Could you check a few things on this drawing? It's one solid part, dimensions in mm from its lowest x, y, z. A direction names the side the tool comes from. Coordinates: 2 decimals unless noted, no trailing zeros. Write each loop counter-clockwise with the first axis right and the second up, starting at its lowest first coordinate (ties: lowest second). Pieces come first, ordered by that corner, then holes.
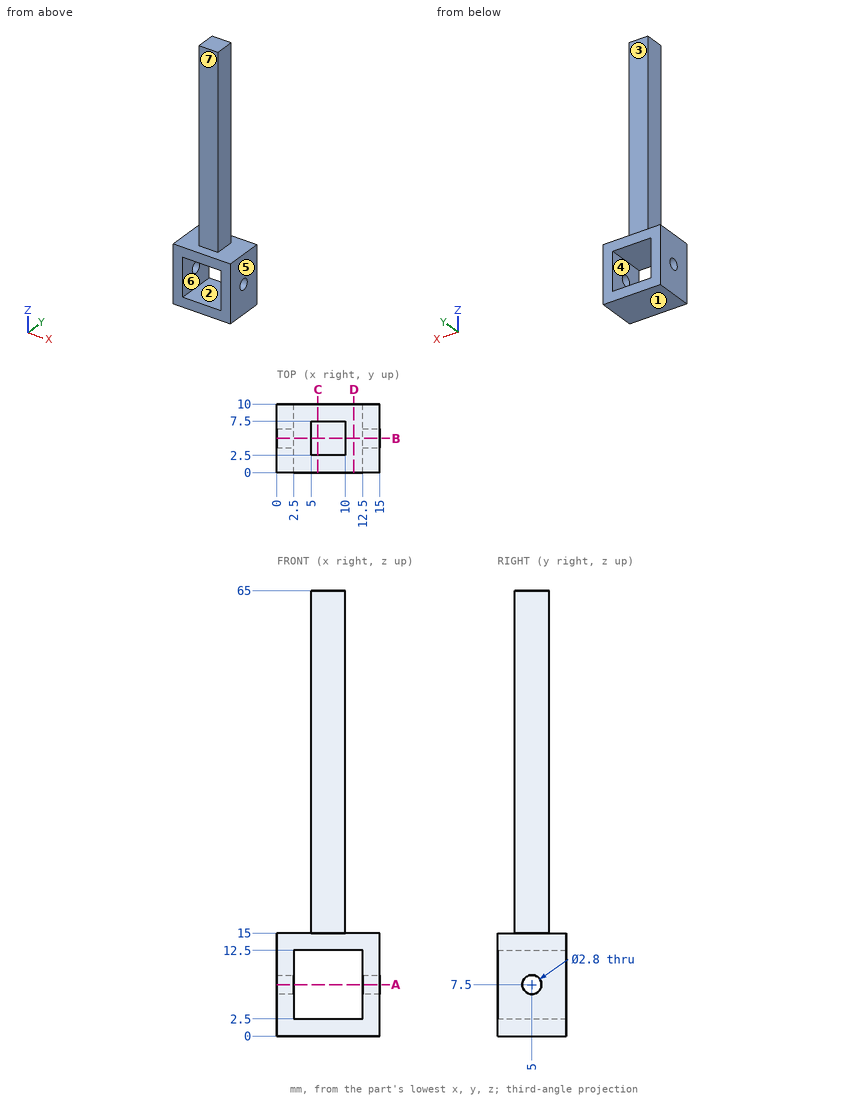
1) Imagine slicing it at A-A on z = 7.5. Please give me the cut outline in (x, y), then the cut area to 3 significant figures.
Values follow:
outline: (0, 0) - (2.5, 0) - (2.5, 3.6) - (0, 3.6) - close; (0, 6.4) - (2.5, 6.4) - (2.5, 10) - (0, 10) - close; (12.5, 0) - (15, 0) - (15, 3.6) - (12.5, 3.6) - close; (12.5, 6.4) - (15, 6.4) - (15, 10) - (12.5, 10) - close
area: 36.0 mm2
2) We'd pull the mould along Z, two halves only. Please class the marked faces 1, 2, 3 and 4: pulls with the +Z half, pulls with the -Z half, needs draft (parallel to the pull), parting line crosses it, or undercut.
Values follow:
face 1: pulls with the -Z half
face 2: undercut
face 3: needs draft
face 4: undercut
3) Imagine slicing it at B-B on y = 5. Please give me the cut outline in (x, z).
Values follow:
outline: (0, 0) - (15, 0) - (15, 6.1) - (12.5, 6.1) - (12.5, 2.5) - (2.5, 2.5) - (2.5, 6.1) - (0, 6.1) - close; (0, 8.9) - (2.5, 8.9) - (2.5, 12.5) - (12.5, 12.5) - (12.5, 8.9) - (15, 8.9) - (15, 15) - (10, 15) - (10, 65) - (5, 65) - (5, 15) - (0, 15) - close
4) On a 3-axis mill with a long thin cutter (end or side, diameter ignored), from which of +Z, -Z, +X, -X, +Y, -Y can I reach the whole of each face in a straight line? I mean the marked faces 5, 6 and 7. Say none if no direction works.
Values follow:
face 5: +Z, -Z, +X, +Y, -Y
face 6: +Y, -Y
face 7: +Z, +X, -X, -Y
5) Imagine slicing it at D-D on x = 11.25. Please give me the cut outline in (y, z).
Values follow:
outline: (0, 0) - (10, 0) - (10, 2.5) - (0, 2.5) - close; (0, 12.5) - (10, 12.5) - (10, 15) - (0, 15) - close
6) Will these pins go through, and if not, where does the flat tip stop? pin 1 (1 mm diameter, centred on x = 9.5, z = 38, fed in from -Y); pin 2 (1.5 mm diameter, centred on y = 5, z = 45.5, fed in from +X); pin 3 (1.5 mm diameter, centred on x = 8, z = 37, fed in from +Y).
Values follow:
pin 1: stops at y = 2.5
pin 2: stops at x = 10
pin 3: stops at y = 7.5
7) I need wall thicknesses on probe 1 along Y at (x, z) = (13.6, 7.5); probe 2 along Z at (x, y) = (14.05, 5); probe 3 along Z at (x, y) = (6.25, 9). Which ranges of each line are inside material? Lowest first, please.
Values follow:
probe 1: y = 0 to 3.6, 6.4 to 10
probe 2: z = 0 to 6.1, 8.9 to 15
probe 3: z = 0 to 2.5, 12.5 to 15
8) Imagine slicing it at C-C on x = 6. Please give me the cut outline in (y, z).
Values follow:
outline: (0, 0) - (10, 0) - (10, 2.5) - (0, 2.5) - close; (0, 12.5) - (10, 12.5) - (10, 15) - (7.5, 15) - (7.5, 65) - (2.5, 65) - (2.5, 15) - (0, 15) - close
